Geometry: final body of the model. Coordinates: model frame, mm. Coordinates: 2 decimals unless noted, no trailing zeros. Loops run counter-clockwise (first coordinate to the right, second up) from the corner with the lowest first, then second, coordinate; pieces in that order, holes last. Notation, with made-up numbers: (54.5, -31) - (107.5, -31) arc R14 cw to (107.5, -12) - close; hole circle Ø8 at (23, -37). An arc over 180 degrees is marked (long way). Put each result on its own line as item: value. Start each with the question number.
1) Draft query along Z for faces 1 (the cylindrical face through (15.77, -9.86, 163.16)), 2 (the flat face through (-1, 0, 56)), 3 (the cylindrical face through (-80.194, -23.574, 108.763)). Return one class per face: +Z half, -Z half, draft (parallel to the pull), parting line (faces both ways), or undercut.
2) Section B-B on y = -14.75. Output: boundary loops of the cut face in (x, z), and give its area (3 significant figures).
3) Contact query for flat-ended pins moving along their axis: pin 1 Ø5 at (y, z) = (-15.5, 111) entering from +X; pin 2 Ø1.5 at (y, z) = (-18.5, 94.5) entering from -X. Output: stop coordinate, or through.
4) Material intervals for line 1 along Z through (x, y) = (0, -12.75); line 2 along X through (y, z) = (-1.5, 118); line 3 along X through (y, z) = (-20.75, 150), sorted ascending. Write a range as from..to.
5) Section A-A on x = 0. Output: boundary loops of the cut face in (y, z), and give its area (3 significant figures).
```python
from build123d import *

# Parameters (mm, degrees)
F0_R     = 29.325687
F1_DEPTH = 25
F2_R     = 5
F3_R     = 5


with BuildPart() as f1:
    # F0 (on Front) → F1 (new body)
    with BuildSketch(Plane.XZ):
        with BuildLine():
            Line((-100, 58.738521), (-100, -41.422263))
            Line((-100, -41.422263), (100, -41.422263))
            Line((100, -41.422263), (100, 58.738521))
            Line((100, 58.738521), (62.691501, 161.250998))
            ThreePointArc((62.691501, 161.250998), (0, 205.149263), (-62.691501, 161.250998))
            Line((-62.691501, 161.250998), (-100, 58.738521))
        make_face()
        with Locations((0, 138.434987)):
            Circle(F0_R, mode=Mode.SUBTRACT)
    extrude(amount=F1_DEPTH)

    # F2
    f2_edges = [f1.edges().sort_by_distance(p)[0] for p in [
        (-29.325687, -25, 138.434987),
    ]]
    fillet(f2_edges, radius=F2_R)

    # F3
    f3_edges = [f1.edges().sort_by_distance(p)[0] for p in [
        (-100, -25, 8.658129),
        (-81.34575, -25, 109.994759),
        (0, -25, 205.149263),
        (100, -25, 8.658129),
        (81.34575, -25, 109.994759),
    ]]
    fillet(f3_edges, radius=F3_R)


solid = f1.part
```
Answer block:
1. face 1: undercut
1. face 2: draft
1. face 3: +Z half
2. outline: (-100, -41.42) - (100, -41.42) - (100, 58.74) - (62.69, 161.25) arc R66.71 ccw to (-62.69, 161.25) - (-100, 58.74) - close; hole circle Ø58.65 at (0, 138.43)
2. area: 38,000 mm²
3. pin 1: stops at x = 81.89
3. pin 2: stops at x = -87.26
4. line 1: z = -41.42..109.11, 167.76..205.15
4. line 2: x = -78.43..-21.03, 21.03..78.43
4. line 3: x = -66.73..-27.01, 27.01..66.73
5. outline: (-25, -41.42) - (0, -41.42) - (0, 109.11) - (-20, 109.11) arc R5 ccw to (-25, 104.11) - close; (-25, 172.76) arc R5 ccw to (-20, 167.76) - (0, 167.76) - (0, 205.15) - (-20, 205.15) arc R5 ccw to (-25, 200.15) - close
5. area: 4,680 mm²
